The drawing under review shows one solid part. Ordinate dimensions are in mm from its lowest x, y, z. A direction names the side the tool comes from. Give positions to 0.01 mm unless a question says otherwise; leave off trailing zeros. Loops run counter-clockwise (first coordinate to the right, second up) from the corner with the lowest first, then second, coordinate; pieces in that order, holes last. Notation, with made-up numbers: (-16.75, -36) - (28.25, -36) arc R27 ccw to (28.25, -2) - close; hole circle Ø2 at (27.5, 4.25). An arc over 180 degrees is marked (long way). One line per item, written item: value. Start each with the question number.
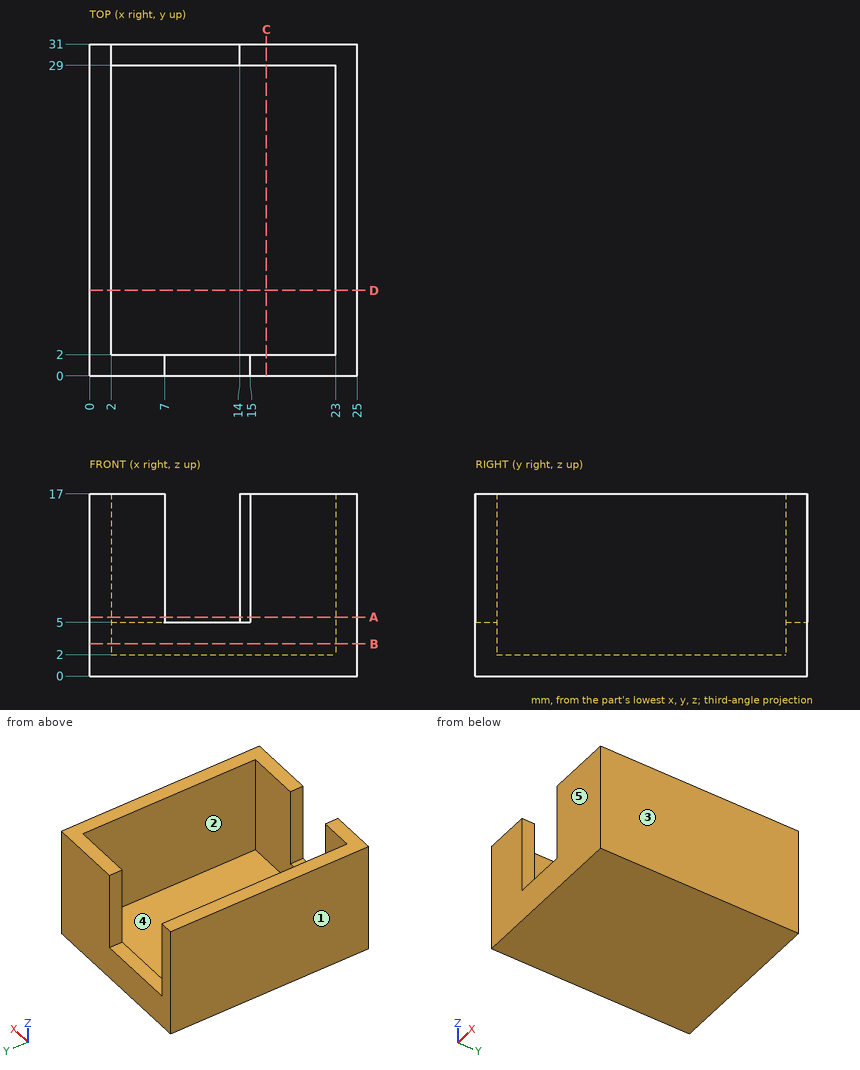
(1) Take a section at B-B on z = 3. State the section outline as (x, y) points, and give its area (3 significant figures).
(2) Machinability: for the marked faces 1 and 2, which of the approach directions +Z, -Z, +X, -X, +Y, -Y give a long, thin tool a straight path to every point of the face, cutting with its end or side? Answer none if there is none.
(3) Take a section at D-D on y = 8. State the section outline as (x, z) points.
(4) For pin 1 Ø10.5 at (x, y) = (10, 14.5) entering from +Z; pin 2 Ø0.6 at (x, y) = (10.5, 1) entering from +Z; pin 3 Ø1.5 at (x, z) = (7, 6.5) entering from +Y, all flat-tipped, find the tip position at first contact; note any pin that passes through.
(5) Take a section at A-A on z = 5.5. State the section outline as (x, y) points, and give its area (3 significant figures).
(6) Take a section at C-C on x = 16.5. State the section outline as (y, z) points.
(7) To check wall thickness, follow L1, parallel to Y at x = 18, z = 16.25; L2, parallel to X at y = 11.5, z = 11; L3, parallel to Z at x = 15.25, y = 16.5. State the ranges of each line that lie inside material, in increasing order. Write a range as from..to.
(8) Draft analysis for pull direction X (two halves, no side actions). For the marked faces 3, 4 and 5, state which applies: pulls with the +X half, pulls with the -X half, needs draft (parallel to the pull), parting line crosses it, or undercut.
Here are the results:
1. outline: (0, 0) - (25, 0) - (25, 31) - (0, 31) - close; hole (2, 2) - (23, 2) - (23, 29) - (2, 29) - close
1. area: 208 mm²
2. face 1: +Z, -Z, -X, +Y, -Y
2. face 2: +Z
3. outline: (0, 0) - (25, 0) - (25, 17) - (23, 17) - (23, 2) - (2, 2) - (2, 17) - (0, 17) - close
4. pin 1: z = 2
4. pin 2: z = 5
4. pin 3: y = 2
5. outline: (0, 0) - (7, 0) - (7, 2) - (2, 2) - (2, 31) - (0, 31) - close; (14, 29) - (23, 29) - (23, 2) - (15, 2) - (15, 0) - (25, 0) - (25, 31) - (14, 31) - close
5. area: 168 mm²
6. outline: (0, 0) - (31, 0) - (31, 17) - (29, 17) - (29, 2) - (2, 2) - (2, 17) - (0, 17) - close
7. L1: 0..2, 29..31
7. L2: 0..2, 23..25
7. L3: 0..2
8. face 3: pulls with the +X half
8. face 4: undercut
8. face 5: needs draft
